CAD build for the part. Positions are in the model's coordinates, mm. Round coordinates to 2 decimals unless told otherwise and drop trailing zeros. Order: outer loops, then holes, each group sorted by start corner. A loop starts at its lowest first (then second) coordinate and runs counter-clockwise, first axis right, second up. Notation, with made-up numbers: M 81,-34 L 106,-34 A25 ccw 106,-19 Z; hole C 70.25,87.5 d6. An arc over 180 degrees is marked long. Answer as a JSON object with one key per item and string values.
Autodesk Inventor part; units mm, degrees
ref_plane "YZ Plane" through (0, 0, 0) normal (1, 0, 0) x (0, 1, 0)
ref_plane "XZ Plane" through (0, 0, 0) normal (0, 1, 0) x (-1, 0, 0)
ref_plane "XY Plane" through (0, 0, 0) normal (0, 0, 1) x (1, 0, 0)
sketch "Sketch1" plane through (0, 0, 0) normal (0, 1, 0) x (-1, 0, 0)
  circle A0 centre (0, 0) radius 85
  dimension "d0" = 170
extrude "Extrusion1" add sketch "Sketch1" along normal blind 15
sketch "Sketch2" plane through (0, 15, 0) normal (0, 1, 0) x (1, 0, 0)
  circle A0 centre (0, 0) radius 85
  line L0 (51, -22.7944) -> (-51, -22.7944)
  line L1 (-56, 50.2056) -> (56, 50.2056)
  line L2 (0, 119) -> (0, -119)
  line L3 (-56, 50.2056) -> (51, -22.7944) construction
  line L4 (56, 50.2056) -> (-51, -22.7944) construction
  line L5 (-56, 50.2056) -> (-51, -22.7944)
  line L6 (56, 50.2056) -> (51, -22.7944)
  line L7 (-119, 0) -> (119, 0)
  point P0 (0, -22.7944)
  point P1 (0, 50.2056)
  point P2 (0, 12)
  dimension "d4" = 112
  dimension "d5" = 73
  dimension "d7" = 102
  dimension "d9" = 12
sketch "Sketch3" plane through (0, 15, 0) normal (0, 1, 0) x (1, 0, 0)
  circle A0 centre (0, 0) radius 76
  point P0 (-76, 0)
  point P1 (76, 0)
  dimension "d10" = 152
hole "Hole1" at (-76, 15, 0) at (76, 15, 0) direction (0, -1, 0) diameter 4.5 depth 15 counterbore diameter 8 counterbore depth 12
properties part number "Build Plate with 35mm FOV Sketch"
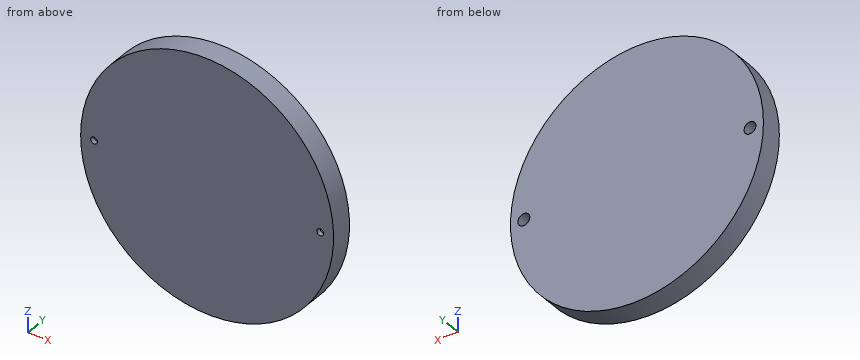
Item 1: Saw through at C-C on y = 8.5. List the corners of the cut face in (x, z), and give its area (3 significant figures).
Worked answers:
{"outline": "C 0,0 d170; hole C -76,0 d8; hole C 76,0 d8", "area": "22,600 mm2"}
Item 2: Saw through at A-A on z = 0. List the corners of the cut face in (x, y).
Worked answers:
{"outline": "M -85,0 L -78.25,0 L -78.25,3 L -80,3 L -80,15 L -85,15 Z; M -73.75,0 L 73.75,0 L 73.75,3 L 72,3 L 72,15 L -72,15 L -72,3 L -73.75,3 Z; M 78.25,0 L 85,0 L 85,15 L 80,15 L 80,3 L 78.25,3 Z"}
Item 3: Drop flat-ended pins along their axis: pin 1 Ø5 at (x, z) = (-76, 0) entering from +Y; pin 2 Ø3 at (y, z) = (1.5, 33.5) entering from -X; pin 3 Ø1.5 at (y, z) = (8, -63.5) entering from +X. Give the stop position or say it passes through.
Worked answers:
{"pin 1": "stops at y = 3", "pin 2": "stops at x = -78.75", "pin 3": "stops at x = 57.34"}
Item 4: Saw through at D-D on z = -70. List the corners of the cut face in (x, y).
Worked answers:
{"outline": "M -48.22,0 L 48.22,0 L 48.22,15 L -48.22,15 Z"}
Item 5: Wall check: line 1 along X through (y, z) = (13.25, -3.5); line 2 along Z through (x, y) = (76, 1); line 3 along Z through (x, y) = (-76, 6.25). Give the ranges that are in metal, low to high. Write a range as [from, to].
Worked answers:
{"line 1": "x = [-84.93, -77.94], [-74.06, 74.06], [77.94, 84.93]", "line 2": "z = [-38.07, -2.25], [2.25, 38.07]", "line 3": "z = [-38.07, -4], [4, 38.07]"}
Item 6: Saw through at B-B on x = -76. List the corners of the cut face in (y, z).
Worked answers:
{"outline": "M 0,-38.07 L 15,-38.07 L 15,-4 L 3,-4 L 3,-2.25 L 0,-2.25 Z; M 0,2.25 L 3,2.25 L 3,4 L 15,4 L 15,38.07 L 0,38.07 Z"}
